The figure shows three views and two pictorial views of one solid part (mm, origin at its lowest corner). Answer the questions. A direction names the side the tool comes from. Coordinates: 2 decimals unless noted, no trailing zeros. Loops run counter-clockwise (first coordinate to the right, second up) from the corner with the lowest first, then second, coordinate; pieces in that order, holes last. Notation, with made-up numbers: M 1.5,36 L 5.5,36 A10 cw 5.5,50 Z; hole C 16,26 d11. An arc over 180 degrees is marked long. Answer in a Markdown table with one row per item. Add a question column.
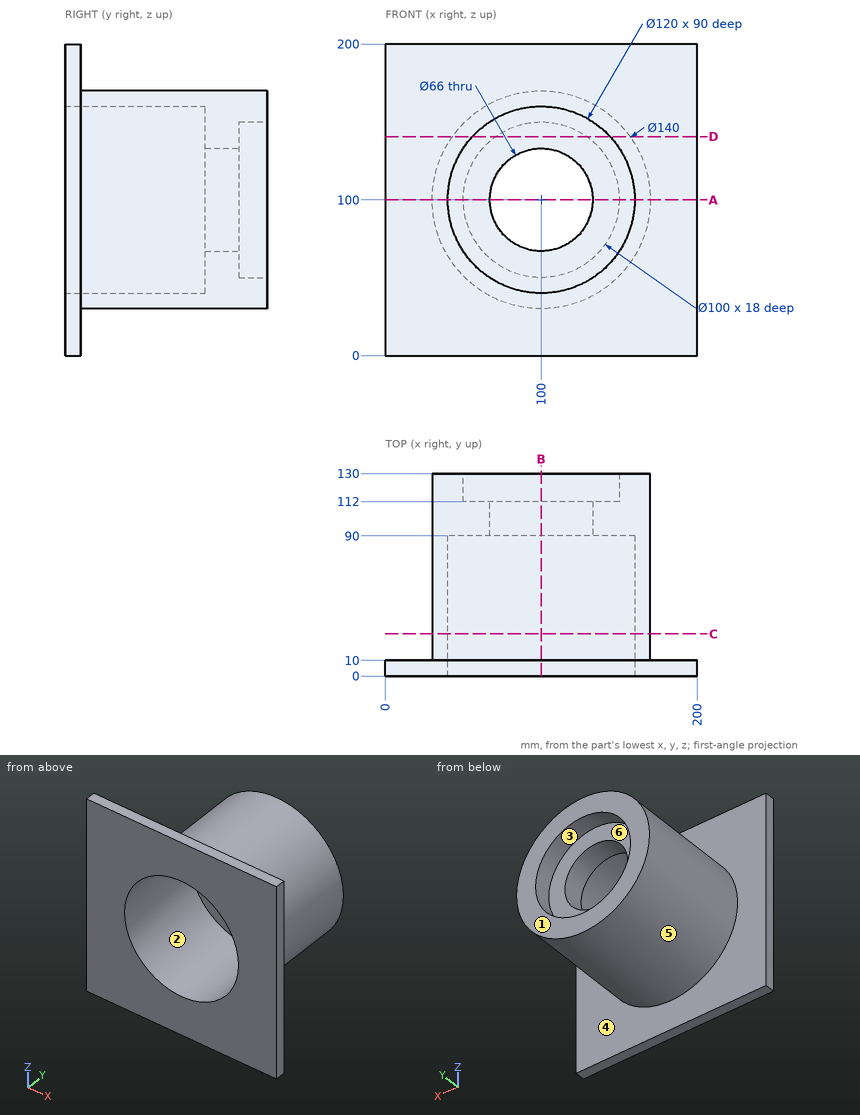
(1) A cutting plane is placed at D-D (z = 140.5). Give the vertices of the cut face in (x, y).
(2) A cutting plane is placed at B-B (x = 100). Give the vertices of the cut face in (y, z), plus the area to 3 significant figures.
(3) For the marked faces 1, 2 and 3, determine the directions among +Z, -Z, +X, -X, +Y, -Y from which every point of the face is accessible in a straight line to the end or side of a thin tool.
(4) A cutting plane is placed at A-A (z = 100). Give the vertices of the cut face in (x, y), plus the area to 3 significant figures.
(5) A cutting plane is placed at C-C (y = 27). Give the vertices of the cut face in (x, z), plus the area to 3 significant figures.
(6) Straight lines are drawn through the part: line 1 (Z direction, x = 97.5, y = 5); line 2 (Z direction, x = 100, y = 51); line 3 (X direction, y = 97, z = 100). For each, find the intervals that lie inside material, in ascending order.
(7) The mould has two halves that part along Z. Classify the marked faces 4, 5 and 6: released by +Z, released by -Z, zero draft, split by the parting line, or undercut.
(8) Each of these flat-tipped pins is pushed along its axis until it touches: pin 1 (1 mm diameter, centred on x = 148, y = 105, fed in from +Z); pin 2 (3 mm diameter, centred on x = 90, z = 170, fed in from -Y); pin 3 (6 mm diameter, centred on x = 58, y = 13.5, fed in from -Z); pin 4 (6 mm diameter, centred on x = 37, z = 31.5, fed in from +Y). Where does it stop, or does it pass through?
Solved:
| question | item | result |
|---|---|---|
| 1 | outline | M 0,0 L 55.73,0 L 55.73,90 L 144.27,90 L 144.27,0 L 200,0 L 200,10 L 157.09,10 L 157.09,130 L 129.32,130 L 129.32,112 L 70.68,112 L 70.68,130 L 42.91,130 L 42.91,10 L 0,10 Z |
| 2 | outline | M 0,0 L 10,0 L 10,30 L 130,30 L 130,50 L 112,50 L 112,67 L 90,67 L 90,40 L 0,40 Z; M 0,160 L 90,160 L 90,133 L 112,133 L 112,150 L 130,150 L 130,170 L 10,170 L 10,200 L 0,200 Z |
| 2 | area | 4,750 mm² |
| 3 | face 1 | +Z, -Z, +X, -X, +Y |
| 3 | face 2 | -Y |
| 3 | face 3 | +Y |
| 4 | outline | M 0,0 L 40,0 L 40,90 L 67,90 L 67,112 L 50,112 L 50,130 L 30,130 L 30,10 L 0,10 Z; M 133,90 L 160,90 L 160,0 L 200,0 L 200,10 L 170,10 L 170,130 L 150,130 L 150,112 L 133,112 Z |
| 4 | area | 4,750 mm² |
| 5 | outline | C 100,100 d140; hole C 100,100 d120 |
| 5 | area | 4,080 mm² |
| 6 | line 1 | z = 0 to 40.05, 159.95 to 200 |
| 6 | line 2 | z = 30 to 40, 160 to 170 |
| 6 | line 3 | x = 30 to 67, 133 to 170 |
| 7 | face 4 | zero draft |
| 7 | face 5 | split by the parting line |
| 7 | face 6 | undercut |
| 8 | pin 1 | stops at z = 151.42 |
| 8 | pin 2 | stops at y = 0 |
| 8 | pin 3 | stops at z = 41.87 |
| 8 | pin 4 | stops at y = 10 |
